Model file for the job. Use its own axes, mm. Face numbers are marked on the shaded views. A direction names the side the tool comes from. Coordinates: 2 decimals unless noted, no trailing zeros. Order: outer loops, then holes, each group sorted by start corner. A loop starts at its lowest first (then second) coordinate and runs counter-clockwise, first axis right, second up. Notation, with made-up numbers: (58, 34) - (75, 34) arc R33 ccw to (75, 65) - close; hole circle Ø6 at (4, -32). An arc over 180 degrees is marked (long way). Put each result on its own line as item: value. Start each with the question number.
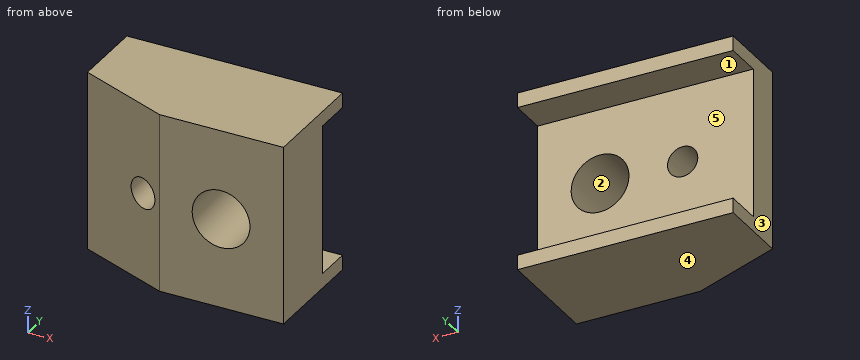
```python
from build123d import *

# Parameters (mm, degrees)
EXTRUDE1_DEPTH            = 19.5
SKETCH2_W                 = 16.3
SKETCH2_H                 = 4.1
CUT_EXTRUDE1_DEPTH        = 33.810059433
M6_3_6_3_DIAMETER_HOLE1_D = 6.3
M4X0_7_TAPPED_HOLE1_D     = 3.3
M4X0_7_TAPPED_HOLE1_DEPTH = 10.1
M4X0_7_TAPPED_HOLE1_TIP   = 0.991420021


with BuildPart() as part:
    # Sketch1 → Extrude1 (new body)
    with BuildSketch(Plane.XY):
        Polygon((-13.5, 0), (-23.5, 4), (-23.5, 12), (0, 12), (0, 0), align=None)
    extrude(amount=EXTRUDE1_DEPTH)

    # Sketch2 → Cut-Extrude1 (cut, through all)
    with BuildSketch(Plane(origin=(0, 0, 0), x_dir=(0, 0, -1), z_dir=(1, 0, 0))):
        with Locations((-9.75, 9.95)):
            Rectangle(SKETCH2_W, SKETCH2_H)
    extrude(amount=-CUT_EXTRUDE1_DEPTH, mode=Mode.SUBTRACT)

    # M6.3 (6.3) Diameter Hole1 (through all)
    with Locations(Plane(origin=(-6.8, 7.9, 9.75), x_dir=(0, 0, 1), z_dir=(0, 1, 0))):
        with Locations((0, 0)):
            Hole(M6_3_6_3_DIAMETER_HOLE1_D / 2)

    # M4x0.7 Tapped Hole1
    with Locations(Plane(origin=(-15.8, 7.9, 9.75), x_dir=(0, 0, 1), z_dir=(0, 1, 0))):
        with Locations((0, 0)):
            Hole(M4X0_7_TAPPED_HOLE1_D / 2, depth=M4X0_7_TAPPED_HOLE1_DEPTH)
            with Locations((0, 0, -(M4X0_7_TAPPED_HOLE1_DEPTH + M4X0_7_TAPPED_HOLE1_TIP / 2))):  # 118° drill point
                Cone(0, M4X0_7_TAPPED_HOLE1_D / 2, M4X0_7_TAPPED_HOLE1_TIP, mode=Mode.SUBTRACT)


solid = part.part
```
Item 1: Pull direction Z, two halves, no side cores. Call the marked faces 3, 4 and 5: pulls with the +Z half, pulls with the -Z half, needs draft (parallel to the pull), parting line crosses it, or undercut.
Item 2: Flat gauge pins, fed straight in: pin 1 Ø2 at (x, z) = (-15.8, 9.75) entering from +Y (3 decimals); pin 2 Ø1.5 at (x, z) = (-5, 5) entering from +Y. Where does each tip first touch, or does it go through?
Item 3: Wall check: line 1 along X through (y, z) = (4.5, 9.75); line 2 along Z through (x, y) = (-21.75, 9.25); line 3 along Z through (x, y) = (-15.8, 4). Give the ranges that are in metal, low to high.
Item 4: Slice it at C-C, the plane y = 10. Give the cut face in (x, z), plus the area to 3 significant figures.
Item 5: Slice it at A-A, the plane x = -6.8. Give the cut face in (y, z).
Item 6: Slice it at B-B, the plane z = 9.75. Give the cut face in (x, y).
Item 7: 3-axis set-ups, long thin cutter, end or side, ignore diameter. For the marked faces 1 and 2: which of +Z, -Z, +X, -X, +Y, -Y reach the whole face in a straight line?
Item 8: Slice it at D-D, the plane x = -15.8. Give the cut face in (y, z).
Here are the results:
1. face 3: needs draft
1. face 4: pulls with the -Z half
1. face 5: undercut
2. pin 1: passes through
2. pin 2: stops at y = 7.9
3. line 1: x = -23.5 to -17.45, -14.15 to -9.95, -3.65 to 0
3. line 2: z = 0 to 1.6, 17.9 to 19.5
3. line 3: z = 0 to 8.1, 11.4 to 19.5
4. outline: (-23.5, 0) - (0, 0) - (0, 1.6) - (-23.5, 1.6) - close; (-23.5, 17.9) - (0, 17.9) - (0, 19.5) - (-23.5, 19.5) - close
4. area: 75.2 mm^2
5. outline: (0, 0) - (12, 0) - (12, 1.6) - (7.9, 1.6) - (7.9, 6.6) - (0, 6.6) - close; (0, 12.9) - (7.9, 12.9) - (7.9, 17.9) - (12, 17.9) - (12, 19.5) - (0, 19.5) - close
6. outline: (-23.5, 4) - (-17.45, 1.58) - (-17.45, 7.9) - (-23.5, 7.9) - close; (-14.15, 0.26) - (-13.5, 0) - (-9.95, 0) - (-9.95, 7.9) - (-14.15, 7.9) - close; (-3.65, 0) - (0, 0) - (0, 7.9) - (-3.65, 7.9) - close
7. face 1: +X, -X, +Y
7. face 2: +Y, -Y
8. outline: (0.92, 0) - (12, 0) - (12, 1.6) - (7.9, 1.6) - (7.9, 8.1) - (0.92, 8.1) - close; (0.92, 11.4) - (7.9, 11.4) - (7.9, 17.9) - (12, 17.9) - (12, 19.5) - (0.92, 19.5) - close
